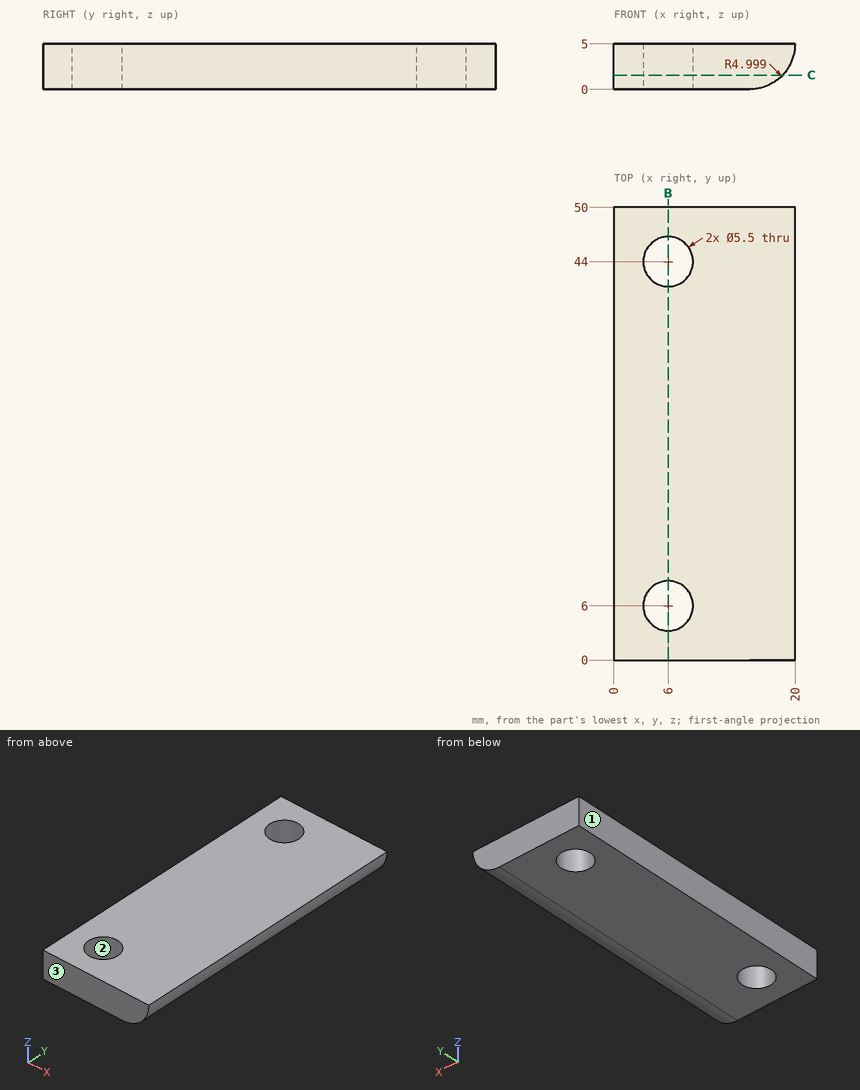
Could you check a few things on this drawing? It's one solid part, dimensions in mm from its lowest x, y, z. Coordinates: 2 decimals unless noted, no trailing zeros. Write each loop counter-clockwise with the first axis right and the second up, starting at its lowest first coordinate (ties: lowest second). Pieces come first, ordered by that corner, then holes. Notation, with made-up numbers: (34.25, 59.25) - (63.25, 59.25) arc R17 ccw to (63.25, 66.25) - close; hole circle Ø7 at (23.25, 6). An arc over 180 degrees is marked (long way). Return JSON: item names as keys, results as strings. Group by question number.
Item 1: Please list where these lines run through material, in increasing order: probe 1 along Y at (x, z) = (6, 0.6); probe 2 along X at (y, z) = (5, 3.5); probe 3 along X at (y, z) = (4, 2.1).
Item 2: I'm going to push a flat-ended pin straight in: pin 1 Ø1.5 at (x, y) = (17.5, 43.5) entering from -Z. Where does the tip first touch, or does it pass through?
Item 3: We'd pull the mould along Y, two halves only. Please class the marked faces 1, 2 and 3: pulls with the +Y half, pulls with the -Y half, needs draft (parallel to the pull), parting line crosses it, or undercut.
Item 4: If we section it at C-C (z = 1.55): Write out the boundary of the cut face in (x, y).
Item 5: If we section it at B-B (x = 6): Write out the boundary of the cut face in (y, z), then the cut area to 3 significant figures.
Return value:
{
 "1": {"probe 1": "y = 0 to 3.25, 8.75 to 41.25, 46.75 to 50", "probe 2": "x = 0 to 3.44, 8.56 to 19.77", "probe 3": "x = 0 to 4.11, 7.89 to 19.07"},
 "2": {"pin 1": "stops at z = 0.32"},
 "3": {"face 1": "needs draft", "face 2": "undercut", "face 3": "pulls with the -Y half"},
 "4": {"outline": "(0, 0) - (18.62, 0) - (18.62, 50) - (0, 50) - close; hole circle Ø5.5 at (6, 6); hole circle Ø5.5 at (6, 44)"},
 "5": {"outline": "(0, 0) - (3.25, 0) - (3.25, 5) - (0, 5) - close; (8.75, 0) - (41.25, 0) - (41.25, 5) - (8.75, 5) - close; (46.75, 0) - (50, 0) - (50, 5) - (46.75, 5) - close", "area": "195 mm^2"}
}
